Geometry: see drawing. Coordinates: mm, zero at the bounding-box minimum. Coordinates: 2 decimals unless noted, no trailing zeros. Loops run counter-clockwise (first coordinate to the right, second up) from the corner with the lowest first, then second, coordinate; pieces in that order, holes last.
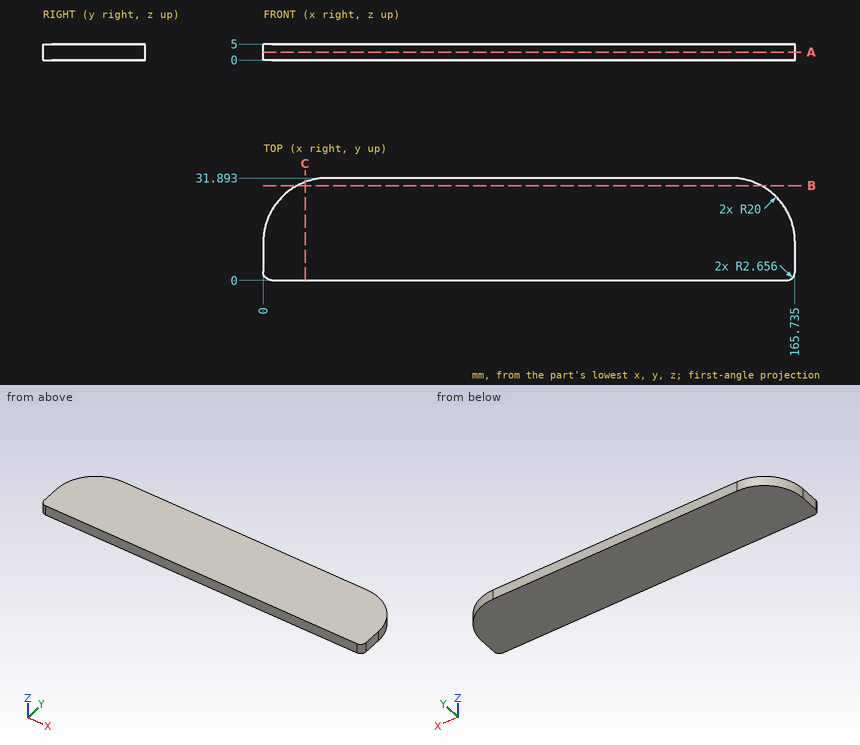
Item 1: Line query: L1, parallel to X at y = 13, z = 3.75 (1 decimal); L2, parallel to X at y = 28, z = 3.8 (1 decimal); L3, parallel to Y at x = 147.5, z = 2.55 (1 decimal). Output: solid intervals per line, ascending.
Result:
L1: x = 0 to 165.7
L2: x = 8.1 to 157.6
L3: y = 0 to 31.8
Item 2: Contact query for flat-ended pins moving along their axis: P1, Ø10, axis at x = 111.5, y = 12, coming from the -Z side; P2, Ø2, axis at y = 26, z = 2.5, coming from the -X side. Output: stop coordinate, or through.
Result:
P1: stops at z = 0
P2: stops at x = 4.89
Item 3: Section query C-C (x = 13). Output: boundary loops of the cut face in (y, z).
Result:
outline: (0, 0) - (30.63, 0) - (30.63, 5) - (0, 5) - close
Item 4: Section query A-A (z = 2.5). Output: boundary loops of the cut face in (x, y) (1 decimal), then the cut area to 3 significant figures.
Result:
outline: (0, 2.7) arc R2.7 ccw to (2.7, 0) - (163.1, 0) arc R2.7 ccw to (165.7, 2.7) - (165.7, 11.9) arc R20 ccw to (145.7, 31.9) - (20, 31.9) arc R20 ccw to (0, 11.9) - close
area: 5,110 mm2
Item 5: Section query B-B (y = 29.5). Output: boundary loops of the cut face in (x, z).
Result:
outline: (10.51, 0) - (155.22, 0) - (155.22, 5) - (10.51, 5) - close
